from build123d import *

# Parameters (mm, degrees)
BOSS_EXTRUDE1_DEPTH      = 30
SKETCH3_R                = 4
CUT_EXTRUDE1_DEPTH       = 40
SKETCH4_W                = 3
SKETCH4_H                = 41
BOSS_EXTRUDE2_DEPTH      = 4
BOSS_EXTRUDE3_DEPTH      = 25
BOSS_EXTRUDE3_DEPTH_BACK = 4
SKETCH5_W                = 3
SKETCH5_H                = 7.75
BOSS_EXTRUDE4_REACH      = 69.734
SKETCH6_W                = 4
SKETCH6_H                = 56.5
CUT_EXTRUDE3_DEPTH       = 47
CUT_EXTRUDE4_DEPTH       = 47


with BuildPart() as part:
    # Sketch1 → Boss-Extrude1 (new body)
    with BuildSketch(Plane(origin=(0, 0, 0), x_dir=(1, 0, 0), z_dir=(0, 1, 0))):
        Polygon((-12.8, -12.8), (-13.1, 12.8), (13.1, 12.8), (12.8, -12.6), (16.799721029, -12.6472408), (17.147523085, 16.8), (-17.147149649, 16.8), (-16.79972537, -12.846871782), align=None)
    extrude(amount=BOSS_EXTRUDE1_DEPTH)

    # Sketch3 → Cut-Extrude1 (cut)
    with BuildSketch(Plane(origin=(16.946733814, 0, 0.200158273), x_dir=(0.011810199887684227, 0, -0.9999302571572745), z_dir=(0.9999302571572745, 0, 0.011810199887684227))):
        with Locations(Location((-0.747950682, 15, 0), (0, 0, 180))):
            Circle(SKETCH3_R)
    extrude(amount=-CUT_EXTRUDE1_DEPTH, mode=Mode.SUBTRACT)

    # Sketch4 → Boss-Extrude2 (add)
    with BuildSketch(Plane(origin=(0, 0, -16.8), x_dir=(-1, 0, 0), z_dir=(0, 0, -1))):
        with Locations((12.499813282, 15)):
            Rectangle(SKETCH4_W, SKETCH4_H)
    extrude(amount=-BOSS_EXTRUDE2_DEPTH)

    # Sketch5 → Boss-Extrude3 (add, two sides: drawn at the far end of the back side and taken through both)
    with BuildSketch(Plane(origin=(0, 0, -16.8), x_dir=(-1, 0, 0), z_dir=(0, 0, -1)).offset(-BOSS_EXTRUDE3_DEPTH_BACK)):
        with Locations((12.499813282, 39.375)):
            Rectangle(SKETCH5_W, SKETCH5_H)
        with Locations((12.499813282, -9.375)):
            Rectangle(SKETCH5_W, SKETCH5_H)
    extrude(amount=BOSS_EXTRUDE3_DEPTH + BOSS_EXTRUDE3_DEPTH_BACK)

    # Boss-Extrude4: up to this plane
    boss_extrude4_end = Plane(origin=(-16.79972537, 30, 12.846871782), z_dir=(0.9999313425206403, 0, -0.01171794542016394))
    # Sketch6 → Boss-Extrude4 (add, up to the surface)
    with BuildSketch(Plane.ZY.offset(13.999813282), mode=Mode.PRIVATE) as boss_extrude4_sk1:
        with Locations((-14.8, 15)):
            Rectangle(SKETCH6_W, SKETCH6_H)
    boss_extrude4_tool1 = split(extrude(boss_extrude4_sk1.sketch, amount=BOSS_EXTRUDE4_REACH, mode=Mode.PRIVATE), bisect_by=boss_extrude4_end, keep=Keep.BOTH, mode=Mode.PRIVATE)
    add(boss_extrude4_tool1.solids().sort_by_distance((-13.999813, 15, -14.8))[0])

    # Sketch7 → Cut-Extrude3 (cut)
    with BuildSketch(Plane(origin=(-16.947947202, 0, 0.198608756), x_dir=(0.01171794542016394, 0, 0.9999313425206403), z_dir=(-0.9999313425206403, 0, 0.01171794542016394))):
        Polygon((15.81172836, 30), (-12.999501269, 30), (-12.999501269, 0), (19.011921217, 0), align=None)
    extrude(amount=-CUT_EXTRUDE3_DEPTH, mode=Mode.SUBTRACT)

    # Sketch8 → Cut-Extrude4 (cut)
    with BuildSketch(Plane(origin=(-0.152327446, 0, -12.998608756), x_dir=(0.9999313425206403, 0, -0.011717945420163944), z_dir=(0.011717945420163944, 0, 0.9999313425206403))):
        Polygon((-10.848230648, 0), (-10.848230648, 46.508852654), (34.891429073, 42.782410239), (32.959466486, 0), (23.967074224, -10.626450369), align=None)
    extrude(amount=-CUT_EXTRUDE4_DEPTH, mode=Mode.SUBTRACT)


solid = part.part
Can you work these out from the model? Positions are in its coordinate system, mm. A direction names the side the tool comes from. Give positions to 0.01 mm unless a question says otherwise; leave off trailing zeros. Order: outer loops, then holes, each group sorted by start corner. A loop starts at its lowest first (then second) coordinate and runs counter-clockwise, first axis right, second up. Notation, with made-up numbers: M -9,30.5 L 6,30.5 A12 ccw 6,48.5 Z; hole C 24,-21 d2. An arc over 180 degrees is marked long. Use one line per item in the form item = value. Start each with the question number.
Item 1: If we section it at D-D (z = -37.75): Write out the boundary of the cut face in (x, y).
Item 2: If we section it at B-B (y = 32): Write out the boundary of the cut face in (x, z), then the cut area to 3 significant figures.
Item 3: For faces 1 (the flat face through (-12, -5.5, -29)), 2 (the flat face through (-14, -9, -29)), 3 (the flat face through (-14, -7, -12.8)), which set-ups out of +Z, -Z, +X, -X, +Y, -Y let a thin tool reach every point of the face, with its end or its side?
Item 4: If I drill on line 1 along Y through (x, z) = (-11.25, -22.5); line 2 along X through (y, z) = (-9, -29); line 3 along Z through (x, y) = (-14.5, 34.5), over which ranges is the centre line in solid material (lowest first)?
Item 5: If we section it at A-A (z = -24): Write out the boundary of the cut face in (x, y).
Item 6: Will these pins go through, and if not, where does the flat tip stop? pin 1 Ø2 at (x, y) = (-11.5, 7.5) entering from +Z; pin 2 Ø1.8 at (x, y) = (-13.5, 7.5) entering from -Z; pin 3 Ø6 at (y, z) = (-8, -33) entering from -X.
Item 7: If we section it at C-C (x = -12.75): Write out the boundary of the cut face in (y, z).
Item 8: We'd pull the mould along Y, two halves only. Please class faces 4 (the flat face through (-13, 43.25, -24)), 5 (the flat face through (-14, 39, -29)), 6 (the flat face through (-13, 35.5, -29)), 7 (the flat face through (-14, 15, -16.8)): +Y half, -Y half, draft (parallel to the pull), parting line (faces both ways), or undercut.
Outcome:
q1.outline = M -14,-13.25 L -11,-13.25 L -11,-5.5 L -14,-5.5 Z; M -14,35.5 L -11.29,35.5 L -11.29,43.25 L -14,43.25 Z
q2.outline = M -17.15,-16.8 L -11.05,-16.8 L -11,-12.87 L -11,-12.8 L -17.1,-12.8 Z
q2.area = 24.4 mm2
q3.face_1 = -Z, +X, -X
q3.face_2 = -Z, -X, +Y, -Y
q3.face_3 = +Z, +X, -X, +Y, -Y
q4.line_1 = -13.25 to -5.5, 35.5 to 43.25
q4.line_2 = -14 to -11
q4.line_3 = -16.8 to -12.8
q5.outline = M -14,-13.25 L -11,-13.25 L -11,-5.5 L -14,-5.5 Z; M -14,35.5 L -11.13,35.5 L -11.13,43.25 L -14,43.25 Z
q6.pin_1 = -12.85
q6.pin_2 = -16.8
q6.pin_3 = -14
q7.outline = M -13.25,-41.8 L -5.5,-41.8 L -5.5,-16.8 L 35.5,-16.8 L 35.5,-41.8 L 43.25,-41.8 L 43.25,-12.8 L 30,-12.8 L 30,-12.85 L 0,-12.85 L 0,-12.8 L -13.25,-12.8 Z
q8.face_4 = +Y half
q8.face_5 = draft
q8.face_6 = undercut
q8.face_7 = undercut
